from build123d import *

# Parameters (mm, degrees)
SKETCH_2_R          = 2.5
EXTRUDE_1_DEPTH     = 29
SKETCH_3_R          = 2.5
EXTRUDE_2_DEPTH     = 26
SKETCH_5_W          = 17
SKETCH_5_H          = 12
SKETCH_5_R          = 1.15
EXTRUDE_4_DEPTH     = 6.5
SKETCH_6_R          = 2
CUT_EXTRUDE_1_DEPTH = 10
SKETCH_7_W          = 12
SKETCH_7_H          = 17
SKETCH_7_R          = 1.15
EXTRUDE_5_DEPTH     = 6.5
SKETCH_8_R          = 2
CUT_EXTRUDE_2_DEPTH = 10


with BuildPart() as part:
    # 스케치1 → 회전1 (revolve)
    with BuildSketch(Plane.XY):
        with BuildLine():
            Line((0, -5), (0, 5))
            ThreePointArc((0, 5), (-5, 0), (0, -5))
        make_face()
    revolve(axis=Axis((0, 7.642806544, 0), (0, -1, 0)))

    # 스케치2 → 보스-돌출1 (add)
    with BuildSketch(Plane(origin=(0, 0, 0), x_dir=(1, 0, 0), z_dir=(0, 1, 0))):
        Circle(SKETCH_2_R)
    extrude(amount=-EXTRUDE_1_DEPTH)

    # 스케치3 → 보스-돌출2 (add)
    with BuildSketch(Plane(origin=(0, 0, 0), x_dir=(0, 0, -1), z_dir=(1, 0, 0))):
        Circle(SKETCH_3_R)
    extrude(amount=-EXTRUDE_2_DEPTH)

    # 스케치5 → 보스-돌출4 (add)
    with BuildSketch(Plane(origin=(0, -35.5, 0), x_dir=(-1, 0, 0), z_dir=(0, -1, 0))):
        Rectangle(SKETCH_5_W, SKETCH_5_H)
        with Locations((0, 3.75)):
            Circle(SKETCH_5_R, mode=Mode.SUBTRACT)
        with Locations((0, -3.75)):
            Circle(SKETCH_5_R, mode=Mode.SUBTRACT)
    extrude(amount=-EXTRUDE_4_DEPTH)

    # 스케치6 → 컷-돌출1 (cut)
    with BuildSketch(Plane(origin=(0, -29, 0), x_dir=(1, 0, 0), z_dir=(0, 1, 0))):
        with Locations((0, 3.75)):
            Circle(SKETCH_6_R)
        with Locations((0, -3.75)):
            Circle(SKETCH_6_R)
    extrude(amount=CUT_EXTRUDE_1_DEPTH, mode=Mode.SUBTRACT)

    # 스케치7 → 보스-돌출5 (add)
    with BuildSketch(Plane(origin=(-32.5, 0, 0), x_dir=(0, 0, -1), z_dir=(1, 0, 0))):
        Rectangle(SKETCH_7_W, SKETCH_7_H)
        with Locations((-3.75, 0)):
            Circle(SKETCH_7_R, mode=Mode.SUBTRACT)
        with Locations((3.75, 0)):
            Circle(SKETCH_7_R, mode=Mode.SUBTRACT)
    extrude(amount=EXTRUDE_5_DEPTH)

    # 스케치8 → 컷-돌출2 (cut)
    with BuildSketch(Plane(origin=(-26, 0, 0), x_dir=(0, 0, -1), z_dir=(1, 0, 0))):
        with Locations((-3.75, 0)):
            Circle(SKETCH_8_R)
        with Locations((3.75, 0)):
            Circle(SKETCH_8_R)
    extrude(amount=CUT_EXTRUDE_2_DEPTH, mode=Mode.SUBTRACT)


solid = part.part
Work out the finished part from the listing and answer in its coordinate system (mm). A direction names the side the tool comes from. Give positions to 0.01 mm unless a question says otherwise; leave off trailing zeros. Loops run counter-clockwise (first coordinate to the right, second up) from the corner with the lowest first, then second, coordinate; pieces in that order, holes last. Notation, with made-up numbers: (25.25, 87) - (56.25, 87) arc R20 ccw to (56.25, 110) - close; hole circle Ø3 at (23.5, 83.5). An arc over 180 degrees is marked (long way). Answer in a Markdown table with one row per item. Add a question column.
Q1. Each of these flat-tipped pins is pushed along its axis until it touches: P1, Ø2, axis at y = -25, z = -4, coming from the +X side; P2, Ø3, axis at y = -16.5, z = -2.5, coming from the +X side; P3, Ø1.4, axis at y = 0, z = -3.75, coming from the -X side; P4, Ø1.4, axis at x = 0, z = 3.75, coming from the +Y side. Where does it stop, or does it pass through?
Q2. A tool of negligible diameter and unlimited length cuts with its end or side. For faces 4 (the flat face through (-8.5, -32, 0)), 5 (the cylindrical face through (0.02, -24.07, 1.75)), 6 (the cylindrical face through (-0.33, -16.49, -2.48)), from which of +Z, -Z, +X, -X, +Y, -Y can it reach the whole face along a straight path? Write none if from no direction.
Q3. The part is cut by section A-A (y = 0). Determine the outline of the cut face in (x, z).
Q4. Determine the mould class of faces 1 (the cylindrical face through (-21.07, 0.02, -1.75)), 2 (the flat face through (-32.5, 0, 0)), 3 (the cylindrical face through (-29.3, 0.05, -2.6)) for opening direction X: released by +X, released by -X, zero draft, split by the parting line, or undercut.
Q5. The part is cut by section D-D (y = -31.5). Determine the outline of the cut face in (x, z).
Q6. Consider line 1 along Y through (x, z) = (-27.5, 3.75); line 2 along X through (y, z) = (2, 3.5). Determine where each line is inside the solid, lowest interval first.
Q7. The part is cut by section B-B (z = -3.75). Determine the outline of the cut face in (x, y).
Q8. The part is cut by section C-C (z = 0). Determine the outline of the cut face in (x, y).
Solution:
| question | item | result |
|---|---|---|
| 1 | P1 | passes through |
| 1 | P2 | stops at x = 2.29 |
| 1 | P3 | stops at x = -3.96 |
| 1 | P4 | stops at y = 3.96 |
| 2 | face 4 | +Z, -Z, -X, -Y |
| 2 | face 5 | +Z |
| 2 | face 6 | none |
| 3 | outline | (-32.5, -6) - (-26, -6) - (-26, -4.9) - (-32.5, -4.9) - close; (-32.5, -2.6) - (-26, -2.6) - (-26, -1.75) - (-16, -1.75) - (-16, -2.5) - (-4.33, -2.5) arc R5 ccw (long way) to (-4.33, 2.5) - (-16, 2.5) - (-16, 1.75) - (-26, 1.75) - (-26, 2.6) - (-32.5, 2.6) - close; (-32.5, 4.9) - (-26, 4.9) - (-26, 6) - (-32.5, 6) - close |
| 4 | face 1 | undercut |
| 4 | face 2 | released by -X |
| 4 | face 3 | zero draft |
| 5 | outline | (-8.5, -6) - (8.5, -6) - (8.5, 6) - (-8.5, 6) - close; hole circle Ø2.3 at (0, -3.75); hole circle Ø2.3 at (0, 3.75) |
| 6 | line 1 | y = -8.5 to -1.15, 1.15 to 8.5 |
| 6 | line 2 | x = -32.5 to -26, -2.96 to 2.96 |
| 7 | outline | (-32.5, -8.5) - (-26, -8.5) - (-26, -1.15) - (-32.5, -1.15) - close; (-32.5, 1.15) - (-26, 1.15) - (-26, 8.5) - (-32.5, 8.5) - close; (-8.5, -35.5) - (-1.15, -35.5) - (-1.15, -29) - (-8.5, -29) - close; circle Ø6.61 at (0, 0); (1.15, -35.5) - (8.5, -35.5) - (8.5, -29) - (1.15, -29) - close |
| 8 | outline | (-32.5, -8.5) - (-26, -8.5) - (-26, -2.5) - (-4.33, -2.5) arc R5 ccw to (-2.5, -4.33) - (-2.5, -29) - (-8.5, -29) - (-8.5, -35.5) - (8.5, -35.5) - (8.5, -29) - (2.5, -29) - (2.5, -4.33) arc R5 ccw (long way) to (-4.33, 2.5) - (-26, 2.5) - (-26, 8.5) - (-32.5, 8.5) - close |
